Can you work these out from the model? Positions are in its coordinate system, mm. Round coordinates to 2 decimals unless told otherwise and drop trailing zeros. Write each loop counter-clockwise with the first axis right and the second up, starting at its lowest first coordinate (ties: lowest second). Pieces come first, ordered by that corner, then holes.
Q1. If we section it at A-A (x = 0): Please give me the cut outline in (y, z).
Q2. Please list where these lines run through material, in increasing order: line 1 along X through (y, z) = (-2.5, -36.07); line 2 along Z through (x, y) = (-30, -7); line 3 along X through (y, z) = (-1.25, 0).
Q3. I'm going to push flat-ended pins straight in: pin 1 Ø4 at (x, z) = (-30, -36.07) entering from +Y; pin 2 Ø6 at (x, z) = (50.1, -36.07) entering from -Y. Where does each tip first touch, or does it pass through?
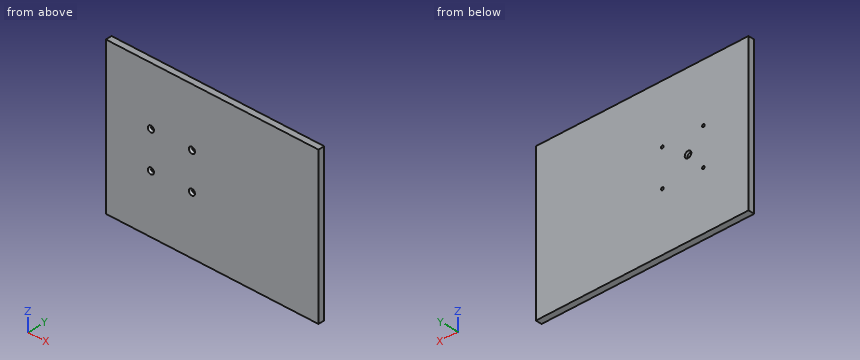
Autodesk Inventor part; units mm, degrees
ref_plane "YZ Plane" through (0, 0, 0) normal (1, 0, 0) x (0, 1, 0)
ref_plane "XZ Plane" through (0, 0, 0) normal (0, 1, 0) x (-1, 0, 0)
ref_plane "XY Plane" through (0, 0, 0) normal (0, 0, 1) x (1, 0, 0)
sketch "Sketch7" plane through (0, 0, 0) normal (0, 1, 0) x (-1, 0, 0)
  line L0 (52.95, -150) -> (-297.05, -150)
  line L1 (-297.05, -150) -> (-297.05, 150)
  line L2 (-297.05, 150) -> (52.95, 150)
  line L3 (52.95, 150) -> (52.95, -150)
  point P0 (0, 0)
  point P1 (52.95, 0)
  dimension "d32" = 350
  dimension "d33" = 300
  dimension "d34" = 52.95
extrude "Extrusion4" add sketch "Sketch7" against normal blind 12
sketch "Sketch8" plane through (0, -12, 0) normal (0, -1, 0) x (1, 0, 0)
  line L0 (54.25, -50.07) -> (54.25, 50.07)
  line L1 (45.95, -50.07) -> (45.95, 50.07)
  line L2 (-34.15, -50.07) -> (-34.15, 50.07)
  line L3 (-25.85, -50.07) -> (-25.85, 50.07)
  line L4 (-34.15, -50.07) -> (-25.85, -50.07)
  line L5 (-34.15, 50.07) -> (-25.85, 50.07)
  line L6 (45.95, 50.07) -> (54.25, 50.07)
  line L7 (45.95, -50.07) -> (54.25, -50.07)
  line L8 (-30, -50.07) -> (-30, 50.07)
  line L9 (50.1, -50.07) -> (50.1, 50.07)
  line L10 (-25.85, 0) -> (45.95, 0)
  point P0 (0, 0)
  point P1 (-30, -36.07)
  point P2 (50.1, -36.07)
  point P3 (-30, 36.07)
  point P4 (50.1, 36.07)
  dimension "d37" = 14
hole "Hole3" at (-30, -12, -36.07) at (50.1, -12, -36.07) at (-30, -12, 36.07) at (50.1, -12, 36.07) direction (0, 1, 0) diameter 5.2 end through all countersink diameter 12 countersink angle 90
sketch "Sketch9" plane through (0, -12, 0) normal (0, -1, 0) x (1, 0, 0)
  line L0 (-52.95, 150) -> (-52.95, -150)
  line L1 (-52.95, 150) -> (-117.95, 150)
  line L2 (-117.95, 150) -> (-117.95, -150)
  line L3 (-117.95, -150) -> (-52.95, -150)
  line L4 (-52.95, -150) -> (-52.95, 150)
  point P0 (0, 0)
  dimension "d45" = 65
extrude "Extrusion5" add sketch "Sketch9" against normal up to surface (12 mm away)
sketch "Sketch10" plane through (0, 0, 0) normal (0, 1, 0) x (1, 0, 0)
  circle A0 centre (0, 0) radius 6.4
  line L0 (-117.95, -150) -> (-117.95, 150)
  point P0 (0, 0)
  point P1 (-117.95, 0)
  dimension "d48" = 117.95
  dimension "d49" = 12.8
extrude "Extrusion6" cut sketch "Sketch10" against normal blind 5.29
equation "\"TransitionRadius\" = BendRadius"
properties part number "base_plates" material "Wood (Birch)"
A:
1. outline: (-12, -150) - (0, -150) - (0, -6.4) - (-5.29, -6.4) - (-5.29, 6.4) - (0, 6.4) - (0, 150) - (-12, 150) - close
2. line 1: x = -117.95 to -32.6, -27.4 to 47.5, 52.7 to 297.05
2. line 2: z = -150 to -38.67, -33.47 to 33.47, 38.67 to 150
2. line 3: x = -117.95 to -6.4, 6.4 to 297.05
3. pin 1: passes through
3. pin 2: stops at y = -9
